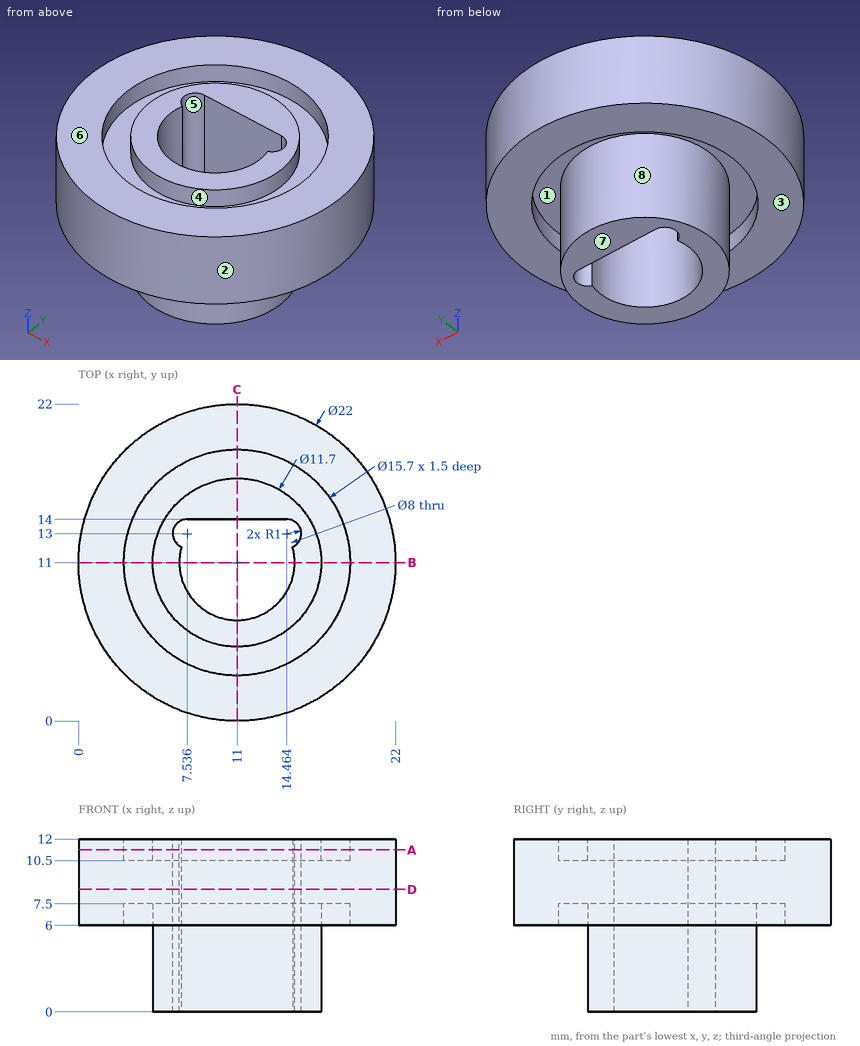
Part print with two shaded views. Sizes in mm from the minimum x, y, z corner. A direction names the side the tool comes from. Round coordinates to 2 decimals unless told otherwise and drop trailing zeros. Order: outer loops, then holes, each group sorted by start corner. A loop starts at its lowest first (then second) coordinate and runs counter-clockwise, first axis right, second up.
(1) 3-axis set-ups, long thin cutter, end or side, ignore diameter. For the marked faces 4, 5, 6, 7 and 8: which of +Z, -Z, +X, -X, +Y, -Y reach the whole face in a straight line?
(2) Drill centre lines: line 1 (X direction, y = 11, z = 11.4); line 2 (X direction, y = 11, z = 9); line 3 (X direction, y = 17.5, z = 11) (1 decimal). Where is each one in solid material? Low to high.
(3) Band-saw the part on B-B (y = 11). List the corners of the cut face in (x, z), then the cut area to 3 significant figures.
(4) Pull direction Y, two halves, no side cores. Call the marked faces 1, 2 and 3: released by +Y, released by -Y, zero draft, split by the parting line, or undercut.
(5) Band-saw the part on A-A (z = 11.25). List the corners of the cut face in (x, y).
(6) Band-saw the part on C-C (x = 11). List the corners of the cut face in (y, z).
(7) Pin check, flat tips, straight feed: pin 1 (2 mm diameter, centred on x = 2, z = 7, fed in from -Y); pin 2 (4 mm diameter, centred on y = 18, z = 7.5, fed in from +X); pin 3 (1 mm diameter, centred on y = 8, z = 1.5, fed in from -X). Stop position of each tip, or through.
(8) Band-saw the part on D-D (z = 8.5). List the corners of the cut face in (x, y), then the cut area to 3 significant figures.
Verdict:
1. face 4: +Z
1. face 5: +Z, -Z
1. face 6: +Z, +X, -X, +Y, -Y
1. face 7: -Z, +X, -X, +Y, -Y
1. face 8: -Z
2. line 1: x = 0 to 3.15, 5.15 to 7, 15 to 16.85, 18.85 to 22
2. line 2: x = 0 to 7, 15 to 22
2. line 3: x = 2.1 to 6.6, 15.4 to 19.9
3. outline: (0, 6) - (3.15, 6) - (3.15, 7.5) - (5.15, 7.5) - (5.15, 0) - (7, 0) - (7, 12) - (5.15, 12) - (5.15, 10.5) - (3.15, 10.5) - (3.15, 12) - (0, 12) - close; (15, 0) - (16.85, 0) - (16.85, 7.5) - (18.85, 7.5) - (18.85, 6) - (22, 6) - (22, 12) - (18.85, 12) - (18.85, 10.5) - (16.85, 10.5) - (16.85, 12) - (15, 12) - close
3. area: 94.2 mm2
4. face 1: undercut
4. face 2: split by the parting line
4. face 3: zero draft
5. outline: circle Ø22 at (11, 11); circle Ø11.7 at (11, 11); hole circle Ø15.7 at (11, 11); hole (7.15, 12.08) arc R4 ccw (long way) to (14.85, 12.08) arc R1 ccw to (14.46, 14) - (7.54, 14) arc R1 ccw to start
6. outline: (0, 6) - (3.15, 6) - (3.15, 7.5) - (5.15, 7.5) - (5.15, 0) - (7, 0) - (7, 12) - (5.15, 12) - (5.15, 10.5) - (3.15, 10.5) - (3.15, 12) - (0, 12) - close; (14, 0) - (16.85, 0) - (16.85, 7.5) - (18.85, 7.5) - (18.85, 6) - (22, 6) - (22, 12) - (18.85, 12) - (18.85, 10.5) - (16.85, 10.5) - (16.85, 12) - (14, 12) - close
7. pin 1: stops at y = 3.45
7. pin 2: stops at x = 20.8
7. pin 3: stops at x = 5.71
8. outline: circle Ø22 at (11, 11); hole (7.15, 12.08) arc R4 ccw (long way) to (14.85, 12.08) arc R1 ccw to (14.46, 14) - (7.54, 14) arc R1 ccw to start
8. area: 330 mm2
